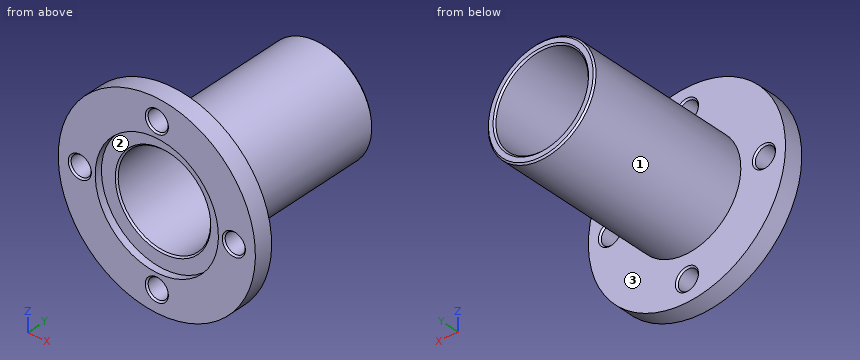
```python
from build123d import *

# Parameters (mm, degrees)
CHAMFER1_SIZE      = 0.5
SKETCH2_R          = 3.25
CUT_EXTRUDE1_DEPTH = 71.455659815
CHAMFER2_SIZE      = 0.5
CHAMFER3_SIZE      = 0.5


with BuildPart() as part:
    # Sketch1 → Revolve1 (revolve)
    with BuildSketch(Plane.XY, mode=Mode.PRIVATE) as revolve1_sk:
        Polygon((-15, 2.3), (-15, 60), (-17.5, 60), (-17.5, 6), (-32, 6), (-32, 0), (-20, 0), (-20, 2.3), align=None)
    revolve(revolve1_sk.sketch.rotate(Axis((0, 0, 0), (0, 1, 0)), 270), axis=Axis((0, 0, 0), (0, 1, 0)))

    # Chamfer1
    chamfer1_edges = [part.edges().sort_by_distance(p)[0] for p in [
        (0, 60, 17.5),
        (0, 60, 15),
    ]]
    chamfer(chamfer1_edges, length=CHAMFER1_SIZE)

    # Sketch2 → Cut-Extrude1 (cut, through all)
    with BuildSketch(Plane(origin=(0, 6, 0), x_dir=(1, 0, 0), z_dir=(0, 1, 0))):
        with Locations(Location((0, 25, 0), (0, 0, 270))):
            Circle(SKETCH2_R)
        with Locations(Location((25, 0, 0), (0, 0, 270))):
            Circle(SKETCH2_R)
        with Locations(Location((0, -25, 0), (0, 0, 270))):
            Circle(SKETCH2_R)
        with Locations(Location((-25, 0, 0), (0, 0, 270))):
            Circle(SKETCH2_R)
    extrude(amount=-CUT_EXTRUDE1_DEPTH, mode=Mode.SUBTRACT)

    # Chamfer2
    chamfer2_edges = [part.edges().sort_by_distance(p)[0] for p in [
        (0, 0, -28.25),
        (0, 6, -28.25),
        (25, 0, -3.25),
        (25, 6, -3.25),
        (0, 0, 21.75),
        (0, 6, 21.75),
        (-25, 0, -3.25),
        (-25, 6, -3.25),
    ]]
    chamfer(chamfer2_edges, length=CHAMFER2_SIZE)

    # Chamfer3
    chamfer3_edges = [part.edges().sort_by_distance(p)[0] for p in [
        (0, 2.3, 15),
    ]]
    chamfer(chamfer3_edges, length=CHAMFER3_SIZE)


solid = part.part
```
The listing builds one solid part. Answer for the finished solid, in the listing's coordinates (mm). Face numbers are marked on the shaded views. Coordinates: 2 decimals unless noted, no trailing zeros. Loops run counter-clockwise (first coordinate to the right, second up) from the corner with the lowest first, then second, coordinate; pieces in that order, holes last. Notation, with made-up numbers: (3, -3) - (31, -3) arc R17 cw to (31, 24) - close; hole circle Ø5 at (-35.75, 3.25). An arc over 180 degrees is marked (long way). Write item = value, one per line.
1) Section C-C (z = 0) is taken. Count the separate pieces of the cut face and the enclosed holes in it, plus the area to 3 significant figures.
Responses:
separate_pieces = 4
enclosed_holes = 0
area = 371 mm^2
2) Section A-A (z = 25) is taken. Determine the outline of the cut face in (x, y).
Responses:
outline = (-19.97, 0) - (-3.75, 0) - (-3.25, 0.5) - (-3.25, 5.5) - (-3.75, 6) - (-19.97, 6) - close; (3.25, 0.5) - (3.75, 0) - (19.97, 0) - (19.97, 6) - (3.75, 6) - (3.25, 5.5) - close
3) Each of these flat-tipped pins is pushed along its axis until it touches: P1, Ø4, axis at y = 27, z = -16, coming from the -X side; P2, Ø8.5, axis at x = 0, z = -25, coming from the -Y side; P3, Ø12, axis at x = 2.5, y = 32, coming from the -Z side; P4, Ø12, axis at x = -2.5, z = -10, coming from the -Y side. Where does it stop, or does it pass through?
Responses:
P1 = -10.5
P2 = 0
P3 = -17.5
P4 = 2.3
4) Find the intervals of material crossed by line 1 along X through (y, z) = (3, 0); line 2 along X through (y, z) = (30, 0); line 3 along Y through (x, z) = (-20, 13), in increasing order.
Responses:
line_1 = -32 to -28.25, -21.75 to -15, 15 to 21.75, 28.25 to 32
line_2 = -17.5 to -15, 15 to 17.5
line_3 = 0 to 6
5) Determine the mould class of the marked faces 1, 2 and 3 for opening direction X: pulls with the +X half, pulls with the -X half, needs draft (parallel to the pull), parting line crosses it, or undercut.
Responses:
face_1 = parting line crosses it
face_2 = undercut
face_3 = needs draft
6) Section B-B (x = -25) is taken. Determine the outline of the cut face in (y, z).
Responses:
outline = (0, -19.97) - (6, -19.97) - (6, -3.75) - (5.5, -3.25) - (0.5, -3.25) - (0, -3.75) - close; (0, 3.75) - (0.5, 3.25) - (5.5, 3.25) - (6, 3.75) - (6, 19.97) - (0, 19.97) - close
7) Section D-D (y = 24.5) is taken. Determine the outline of the cut face in (x, z), plus the area to 3 significant figures.
Responses:
outline = circle Ø35 at (0, 0); hole circle Ø30 at (0, 0)
area = 255 mm^2
